Source: CAD feature listing. Evaluate the final solid. Frame: model axes, mm. A direction names the side the tool comes from. Round coordinates to 2 decimals unless told otherwise and drop trailing zeros. Loops run counter-clockwise (first coordinate to the right, second up) from the corner with the lowest first, then second, coordinate; pieces in that order, holes last. Notation, with made-up numbers: (20, 0) - (24, 0) arc R29 cw to (24, 37) - close; hole circle Ø6 at (87.25, 51.25). An arc over 180 degrees is marked (long way). Write item = value, one per line. Start each with the question number.
Autodesk Inventor part; units mm, degrees
ref_plane "Work Plane2" through (-20.066, 24.7794, 0) normal (0, 0, 1) x (1, 0, 0)
ref_plane "YZ Plane" through (0, 0, 0) normal (1, 0, 0) x (0, 1, 0)
ref_plane "XZ Plane" through (0, 0, 0) normal (0, 1, 0) x (-1, 0, 0)
ref_plane "Work Plane1" through (0, 37.4307, 11.591) normal (0, 0, 1) x (1, 0, 0)
sketch "Sketch1" plane through (0, 37.4307, 11.591) normal (0, 0, 1) x (1, 0, 0)
  circle A0 centre (0, 0) radius 1.2261 construction
  line L0 (4.85, 4.85) -> (-4.85, 4.85) construction
  line L1 (-4.85, 4.85) -> (-4.85, -4.85) construction
  line L2 (-4.85, -4.85) -> (4.85, -4.85) construction
  line L3 (4.85, -4.85) -> (4.85, 4.85) construction
  line L4 (5.85, 5.85) -> (-5.85, 5.85)
  line L5 (-5.85, 5.85) -> (-5.85, -5.85)
  line L6 (-5.85, -5.85) -> (5.85, -5.85)
  line L7 (5.85, -5.85) -> (5.85, 5.85)
  line L8 (20.32, 25.4487) -> (20.32, -10.6193)
  line L9 (-20.32, -10.6193) -> (-20.32, 25.4487)
  line L10 (5.85, 5.85) -> (20.32, 5.85)
  line L11 (20.32, 5.85) -> (20.32, -5.85)
  line L12 (20.32, -5.85) -> (5.85, -5.85)
  line L13 (5.85, -5.85) -> (5.85, 5.85)
  line L14 (-5.85, 5.85) -> (-20.32, 5.85)
  line L15 (-20.32, 5.85) -> (-20.32, -5.85)
  line L16 (-20.32, -5.85) -> (-5.85, -5.85)
  line L17 (-5.85, -5.85) -> (-5.85, 5.85)
  line L18 (18.034, -12.9053) -> (-18.034, -12.9053)
  line L19 (20.32, -5.85) -> (-20.32, -5.85)
  line L20 (-20.32, -5.85) -> (-20.32, -12.9053)
  line L21 (-20.32, -12.9053) -> (20.32, -12.9053)
  line L22 (20.32, -12.9053) -> (20.32, -5.85)
  point P0 (0, -37.4307)
  dimension "d0" = 1
ref_plane "Work Plane2" through (-20.066, 24.7794, 0) normal (0, 0, 1) x (1, 0, 0)
extrude "Extrusion1" add sketch "Sketch1" against normal blind 3 contours L10 L8 L12 L7 | L5 L16 L9 L14 | L12 L8 L22 L21 L18 L20 L9 L16 L6
sketch "Sketch2" plane through (20.32, 24.5254, 11.591) normal (0, 0, -1) x (-1, 0, 0)
  circle A0 centre (35.32, 5.32) radius 3.0099
  circle A1 centre (5.32, 5.32) radius 3.0099
  circle A2 centre (35.32, 5.32) radius 3.2639
  circle A3 centre (5.32, 5.32) radius 3.2639
extrude "Extrusion2" cut sketch "Sketch2" along normal through all contours A0 | A1 | A2 | A3
sketch "Sketch9" plane through (0, 37.4307, 8.591) normal (0, 0, -1) x (-1, 0, 0)
  line L0 (5.85, -5.85) -> (-5.85, -5.85)
  circle A0 centre (-15, -7.5852) radius 3.2639
  line L1 (-20.32, 5.85) -> (-20.32, -12.9053)
  line L2 (-20.32, -12.9053) -> (20.32, -12.9053)
  line L3 (20.32, -12.9053) -> (20.32, 5.85)
  circle A1 centre (15, -7.5852) radius 3.2639
  line L4 (-5.85, 5.85) -> (-20.32, 5.85)
  line L5 (20.32, 5.85) -> (5.85, 5.85)
  line L6 (5.85, 5.85) -> (5.85, -5.85)
  line L7 (-5.85, -5.85) -> (-5.85, 5.85)
  line L8 (20.32, 5.85) -> (20.32, -12.9053)
  line L9 (20.32, 5.85) -> (5.85, 5.85)
  line L10 (20.32, -12.9053) -> (10.32, -12.9053)
  line L11 (10.32, -12.9053) -> (10.32, 5.85)
  line L12 (10.32, 5.85) -> (20.32, 5.85)
  line L13 (20.32, 5.85) -> (20.32, -12.9053)
  line L14 (-20.32, -12.9053) -> (-10.32, -12.9053)
  line L15 (-10.32, -12.9053) -> (-10.32, 5.85)
  line L16 (-10.32, 5.85) -> (-20.32, 5.85)
  line L17 (-20.32, 5.85) -> (-20.32, -12.9053)
  point P0 (0, -37.4307)
  dimension "d36" = 10
  dimension "d37" = 10
extrude "Extrusion9" add sketch "Sketch9" along normal blind 4 contours L5 L3 L2 L11 | L15 L2 L1 L4
sketch "Sketch10" plane through (-20.32, 24.5254, 11.591) normal (0, -1, 0) x (1, 0, 0)
  line L0 (0, 0) -> (40.64, 0)
  line L1 (0, 0) -> (0, -7)
  line L2 (10, -7) -> (0, -7)
  line L3 (10, -3) -> (10, -7)
  line L4 (30.64, -3) -> (10, -3)
  line L5 (30.64, -3) -> (30.64, -7)
  line L6 (40.64, -7) -> (30.64, -7)
  line L7 (40.64, 0) -> (40.64, -7)
  point P0 (20.32, -11.591)
extrude "Extrusion10" add sketch "Sketch10" along normal blind 2
sketch "Sketch11" plane through (0, 37.4307, 11.591) normal (0, 0, 1) x (1, 0, 0)
  circle A0 centre (-40.9999, 4.4119) radius 1
  circle A1 centre (-19.4999, -11.0881) radius 1
  circle A2 centre (-12.9999, 9.4119) radius 1
  circle A3 centre (-10.5, -7.6734) radius 1
  circle A4 centre (-17, 12.8266) radius 1
  circle A5 centre (11, 7.8266) radius 1
  point P0 (6.3071, -26.4348)
  point P1 (13.066, -0.8064)
hole "Hole1" at (13.066, 36.6243, 11.591) at (6.3071, 10.9959, 11.591) at (-40.9999, 41.8426, 11.591) at (-19.4999, 26.3426, 11.591) at (-10.5, 29.7573, 11.591) direction (0, 0, -1) diameter 1.5 end through all
sketch "Sketch12" plane through (-20.32, 22.5254, 11.591) normal (0, -1, 0) x (1, 0, 0)
  line L0 (40.64, 0) -> (0, 0)
  line L1 (0, 0) -> (0, -7)
  line L2 (0, -7) -> (10, -7)
  line L3 (10, -7) -> (10, -3)
  line L4 (10, -3) -> (30.64, -3)
  line L5 (30.64, -3) -> (30.64, -7)
  line L6 (30.64, -7) -> (40.64, -7)
  line L7 (40.64, -7) -> (40.64, 0)
  line L8 (40.64, 0) -> (26.17, 0)
  line L9 (28.64, 0) -> (12, 0)
  line L10 (12, 0) -> (12, -1)
  line L11 (12, -1) -> (28.64, -1)
  line L12 (28.64, -1) -> (28.64, 0)
  point P0 (20.32, -11.591)
  dimension "d49" = 1
  dimension "d52" = 2
  dimension "d53" = 2
extrude "Extrusion11" cut sketch "Sketch12" against normal through all contours L12 L11 L10 L0
properties part number "20_Adapter_Bluray_KES400_Lens_Thorlabs"
(1) Mould query, pull axis Y, two halves, no side actions, for faces 1 (the face through (-15, 43.281, 8)), 2 (the face through (-5.85, 38, 10)), 3 (the face through (13.731, 36.278, 8.042)). Classes: +Y half, -Y half, draft (parallel to the pull), parting line (faces both ways), or undercut.
(2) Pin query (flat end, axial travel): P1, Ø1.4, axis at x = 13.07, y = 36.62, coming from the +Z side; P2, Ø8.5, axis at x = 4, y = 32.5, coming from the +Z side; P3, Ø1, axis at x = 6.5, y = 30, coming from the -Z side. Return the tip coordinate at first contact, or that it passes through.
(3) Cut plane B-B (y = 24.25). Output: boundary loops of the cut face in (x, z).
(4) Material intervals for line 1 along X through (y, z) = (33.25, 7.25); line 2 along X through (y, z) = (42, 11.25); line 3 along Y through (x, z) = (15, 9.75), sorted ascending. Write a range as from..to.
(5) Cut plane A-A (z = 5.75). Output: boundary loops of the cut face in (x, y).
(6) Access query for faces 4 (the face through (0, 31, 8.591)), 5 (the face through (20.32, 33, 8)), 6 (the face through (0, 31.581, 10)), 7 (the face through (8.32, 33, 11)). Directions: +Z, -Z, +X, -X, +Y, -Y. A direction counts if a zero-diameter tool reaches every point of the face in a straight line with its end or side. Return the directions, or none.
(7) Cut plane D-D (y = 36.25). Output: boundary loops of the cut face in (x, z), and give its area (3 significant figures).
Solution:
q1.face_1 = +Y half
q1.face_2 = draft
q1.face_3 = undercut
q2.P1 = through
q2.P2 = 10.59
q2.P3 = 8.59
q3.outline = (-20.32, 4.59) - (-10.32, 4.59) - (-10.32, 8.59) - (10.32, 8.59) - (10.32, 4.59) - (20.32, 4.59) - (20.32, 11.59) - (8.32, 11.59) - (8.32, 10.59) - (-8.32, 10.59) - (-8.32, 11.59) - (-20.32, 11.59) - close
q4.line_1 = -20.32..-10.32, 10.32..20.32
q4.line_2 = -20.32..-8.32, 8.32..20.32
q4.line_3 = 22.53..26.58, 33.11..43.28
q5.outline = (-20.32, 22.53) - (-10.32, 22.53) - (-10.32, 29.03) arc R0.75 cw (long way) to (-10.32, 30.49) - (-10.32, 43.28) - (-20.32, 43.28) - close; (10.32, 22.53) - (20.32, 22.53) - (20.32, 43.28) - (10.32, 43.28) - close; hole circle Ø1.5 at (-19.5, 26.34); hole circle Ø6.53 at (-15, 29.85); hole circle Ø6.53 at (15, 29.85); hole circle Ø1.5 at (13.07, 36.62)
q6.face_4 = -Z, +Y, -Y
q6.face_5 = +Z, -Z, +X, +Y, -Y
q6.face_6 = +Z, -Z, +Y
q6.face_7 = +Z, +Y, -Y
q7.outline = (-20.32, 4.59) - (-10.32, 4.59) - (-10.32, 8.59) - (-5.85, 8.59) - (-5.85, 10.59) - (-8.32, 10.59) - (-8.32, 11.59) - (-20.32, 11.59) - close; (5.85, 8.59) - (10.32, 8.59) - (10.32, 4.59) - (12.42, 4.59) - (12.42, 11.59) - (8.32, 11.59) - (8.32, 10.59) - (5.85, 10.59) - close; (13.72, 4.59) - (20.32, 4.59) - (20.32, 11.59) - (13.72, 11.59) - close
q7.area = 153 mm^2
